Part model, mm, in its own coordinate system. Face numbers are marked on the shaded views. A direction names the side the tool comes from. Give positions to 0.01 mm unless a question says otherwise; leave off trailing zeros. Loops run counter-clockwise (first coordinate to the right, second up) from the corner with the lowest first, then second, coordinate; pieces in that order, holes last. Notation, with made-up numbers: M 29,69 L 46,69 A35 cw 46,104 Z; hole C -23.75,81 d7. An arc over 180 degrees is marked long. Answer in a Markdown table with one row per item.
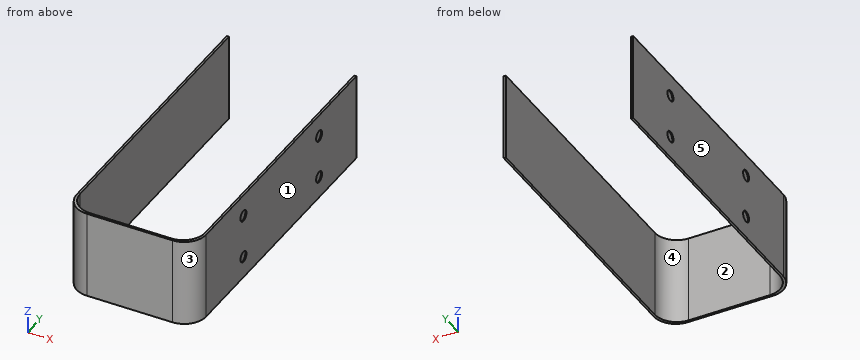
from build123d import *

# Parameters (mm, degrees)
DODANIE_WYCI_GNI_CIE1_DEPTH = 8
SZKIC2_R                    = 0.5
WYTNIJ_WYCI_GNI_CIE1_DEPTH  = 0.1
SZKIC3_R                    = 0.5
WYTNIJ_WYCI_GNI_CIE2_DEPTH  = 0.1


with BuildPart() as part:
    # Szkic1 → Dodanie-wyciągnięcie1 (new body)
    with BuildSketch(Plane.XY):
        with BuildLine():
            Line((-55.680131723, 42.864285714), (-55.680131723, 17.864285714))
            ThreePointArc((-55.680131723, 17.864285714), (-55.094345286, 16.450072152), (-53.680131723, 15.864285714))
            Line((-53.680131723, 15.864285714), (-46.280131723, 15.864285714))
            ThreePointArc((-46.280131723, 15.864285714), (-44.865918161, 16.450072152), (-44.280131723, 17.864285714))
            Line((-44.280131723, 17.864285714), (-44.280131723, 42.864285714))
            Line((-44.280131723, 42.864285714), (-44.080131723, 42.864285714))
            Line((-44.080131723, 42.864285714), (-44.080131723, 17.664285714))
            ThreePointArc((-44.080131723, 17.664285714), (-44.665918161, 16.250072152), (-46.080131723, 15.664285714))
            Line((-46.080131723, 15.664285714), (-53.880131723, 15.664285714))
            ThreePointArc((-53.880131723, 15.664285714), (-55.294345286, 16.250072152), (-55.880131723, 17.664285714))
            Line((-55.880131723, 17.664285714), (-55.880131723, 42.864285714))
            Line((-55.880131723, 42.864285714), (-55.680131723, 42.864285714))
        make_face()
    extrude(amount=DODANIE_WYCI_GNI_CIE1_DEPTH)

    # Szkic2 → Wytnij-wyciągnięcie1 (cut)
    with BuildSketch(Plane(origin=(-44.080131723, 0, 0), x_dir=(0, 0, -1), z_dir=(1, 0, 0))):
        with Locations((-2, 36.614285714)):
            Circle(SZKIC2_R)
        with Locations((-6, 36.614285714)):
            Circle(SZKIC2_R)
        with Locations((-6, 23.914285714)):
            Circle(SZKIC2_R)
        with Locations((-2, 23.914285714)):
            Circle(SZKIC2_R)
    extrude(amount=-WYTNIJ_WYCI_GNI_CIE1_DEPTH, mode=Mode.SUBTRACT)

    # Szkic3 → Wytnij-wyciągnięcie2 (cut)
    with BuildSketch(Plane.ZY.offset(55.880131723)):
        with Locations((2, 36.614285714)):
            Circle(SZKIC3_R)
        with Locations((6, 36.614285714)):
            Circle(SZKIC3_R)
        with Locations((6, 23.914285714)):
            Circle(SZKIC3_R)
        with Locations((2, 23.914285714)):
            Circle(SZKIC3_R)
    extrude(amount=-WYTNIJ_WYCI_GNI_CIE2_DEPTH, mode=Mode.SUBTRACT)


solid = part.part
(1) Pin check, flat tips, straight feed: pin 1 Ø1.1 at (y, z) = (24, 6) entering from -X; pin 2 Ø3 at (x, y) = (-54, 21) entering from -Z; pin 3 Ø0.5 at (y, z) = (24, 2) entering from -X; pin 4 Ø0.5 at (y, z) = (24, 6) entering from +X. Stop position of each tip, or through.
Recorded:
| item | result |
|---|---|
| pin 1 | stops at x = -55.88 |
| pin 2 | passes through |
| pin 3 | stops at x = -55.78 |
| pin 4 | stops at x = -44.18 |
(2) Which spindle directions (+Z, -Z, +X, -X, +Y, -Y) get a long thin tool onto all of the face, cutting with end or side? Do the marked faces 1 and 2. Say none if no direction does.
Recorded:
| item | result |
|---|---|
| face 1 | +Z, -Z, +X, +Y, -Y |
| face 2 | +Z, -Z, +Y |
(3) Saw through at C-C (x = -48.5). Write the cut outline in (y, z), plus the area to 3 significant figures.
Recorded:
| item | result |
|---|---|
| outline | M 15.66,0 L 15.86,0 L 15.86,8 L 15.66,8 Z |
| area | 1.60 mm^2 |
(4) Pull direction X, two halves, no side cores. Call the marked faces 3, 4 and 5: +X half, -X half, draft (parallel to the pull), parting line (faces both ways), or undercut.
Recorded:
| item | result |
|---|---|
| face 3 | +X half |
| face 4 | undercut |
| face 5 | -X half |
(5) Drill centre lines: line 1 along X through (y, z) = (20.5, 1.5); line 2 along Y through (x, z) = (-48.5, 5.25); line 3 along Y through (x, z) = (-44.75, 1.25). Where is each one in solid material? Low to high.
Recorded:
| item | result |
|---|---|
| line 1 | x = -55.88 to -55.68, -44.28 to -44.08 |
| line 2 | y = 15.66 to 15.86 |
| line 3 | y = 16.17 to 16.58 |
(6) Saw through at A-A (y = 23). Write the cut outline in (x, z), plus the area to 3 significant figures.
Recorded:
| item | result |
|---|---|
| outline | M -55.88,0 L -55.68,0 L -55.68,8 L -55.88,8 Z; M -44.28,0 L -44.08,0 L -44.08,8 L -44.28,8 Z |
| area | 3.20 mm^2 |
(7) Saw through at B-B (z = 2). Write the cut outline in (x, y), plus the area to 3 significant figures.
Recorded:
| item | result |
|---|---|
| outline | M -55.88,17.66 A2 ccw -53.88,15.66 L -46.08,15.66 A2 ccw -44.08,17.66 L -44.08,23.41 L -44.18,23.41 L -44.18,24.41 L -44.08,24.41 L -44.08,36.11 L -44.18,36.11 L -44.18,37.11 L -44.08,37.11 L -44.08,42.86 L -44.28,42.86 L -44.28,17.86 A2 cw -46.28,15.86 L -53.68,15.86 A2 cw -55.68,17.86 L -55.68,42.86 L -55.88,42.86 L -55.88,37.11 L -55.78,37.11 L -55.78,36.11 L -55.88,36.11 L -55.88,24.41 L -55.78,24.41 L -55.78,23.41 L -55.88,23.41 Z |
| area | 12.8 mm^2 |
(8) Saw through at D-D (z = 7.5). Write the cut outline in (x, y).
Recorded:
| item | result |
|---|---|
| outline | M -55.88,17.66 A2 ccw -53.88,15.66 L -46.08,15.66 A2 ccw -44.08,17.66 L -44.08,42.86 L -44.28,42.86 L -44.28,17.86 A2 cw -46.28,15.86 L -53.68,15.86 A2 cw -55.68,17.86 L -55.68,42.86 L -55.88,42.86 Z |
